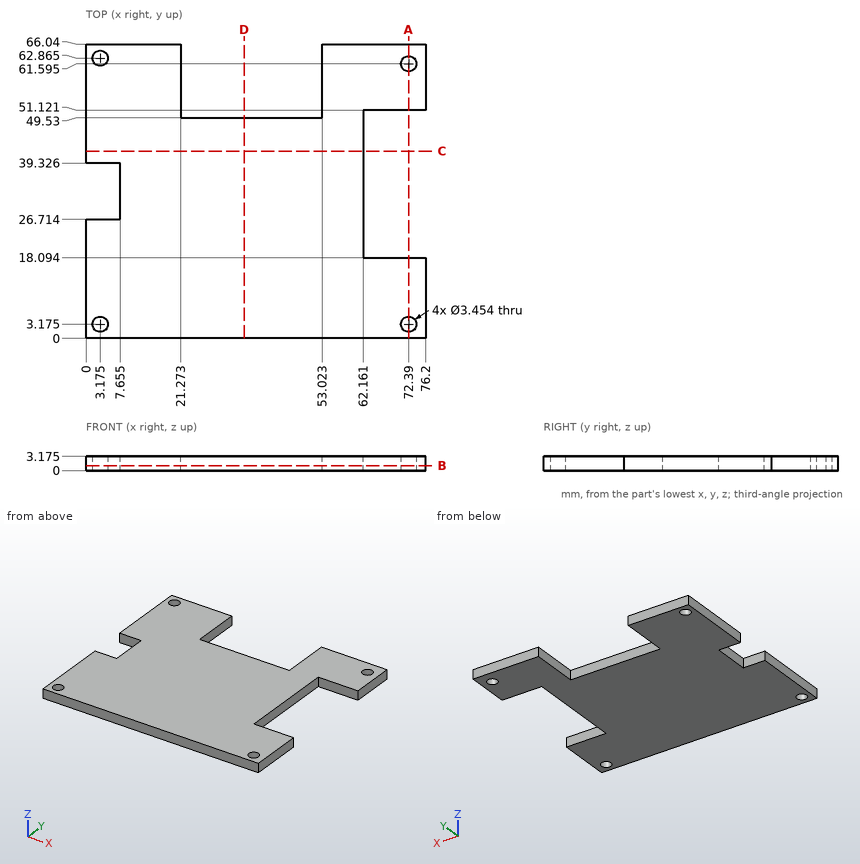
For this review, use the dimensioned drawing (mm, ordinates from the lowest corner) and the shaded views. Give positions to 0.01 mm unless a question says otherwise; leave off trailing zeros. Order: outer loops, then holes, each group sorted by start corner. A loop starts at its lowest first (then second) coordinate and runs counter-clockwise, first axis right, second up. Notation, with made-up numbers: M 25,79.25 L 74,79.25 A11 cw 74,87.25 Z; hole C -12,4.25 d4. An arc over 180 degrees is marked long. One line per question, with ' | ' between items. Start each with the question number.
1) Clearance check with flat-ended pins moving along their axes: P1, Ø3, axis at x = 3.175, y = 62.865, coming from the +Z side; P2, Ø1, axis at y = 32.5, z = 2, coming from the -X side (1 decimal). State where each tip first meets the part, or that it passes through.
2) Consider section D-D, the plane x = 35.5. Give the boundary of the cut face in (y, z) (1 decimal).
3) Consider section A-A, the plane x = 72.39. Give the boundary of the cut face in (y, z) (1 decimal).
4) Consider section B-B, the plane z = 1.1. Give the boundary of the cut face in (x, y) (1 decimal), then the cut area to 3 significant figures.
5) Consider section C-C, the plane y = 42. Give the boundary of the cut face in (x, z) (1 decimal), then the cut area to 3 significant figures.
6) Wall thickness on L1, parallel to Y at x = 72.39, z = 1.2; L2, parallel to Y at x = 7.5, z = 2.65 (1 decimal); L3, parallel to Y at x = 72, z = 1.7 (1 decimal): over which ranges is each line inside the solid? List them lowest first. Write a range as from..to.
Found:
1) P1: passes through | P2: stops at x = 7.7
2) outline: M 0,0 L 49.5,0 L 49.5,3.2 L 0,3.2 Z
3) outline: M 0,0 L 1.4,0 L 1.4,3.2 L 0,3.2 Z; M 4.9,0 L 18.1,0 L 18.1,3.2 L 4.9,3.2 Z; M 51.1,0 L 59.9,0 L 59.9,3.2 L 51.1,3.2 Z; M 63.3,0 L 66,0 L 66,3.2 L 63.3,3.2 Z
4) outline: M 0,0 L 76.2,0 L 76.2,18.1 L 62.2,18.1 L 62.2,51.1 L 76.2,51.1 L 76.2,66 L 53,66 L 53,49.5 L 21.3,49.5 L 21.3,66 L 0,66 L 0,39.3 L 7.7,39.3 L 7.7,26.7 L 0,26.7 Z; hole C 3.2,3.2 d3.5; hole C 3.2,62.9 d3.5; hole C 72.4,3.2 d3.5; hole C 72.4,61.6 d3.5 | area: 3,910 mm²
5) outline: M 0,0 L 62.2,0 L 62.2,3.2 L 0,3.2 Z | area: 197 mm²
6) L1: y = 0..1.45, 4.9..18.09, 51.12..59.87, 63.32..66.04 | L2: y = 0..26.7, 39.3..66 | L3: y = 0..1.5, 4.9..18.1, 51.1..59.9, 63.3..66
